Source: CAD feature listing. Evaluate the final solid. Frame: model axes, mm. A direction names the side the tool comes from. Round coordinates to 2 decimals unless told otherwise and drop trailing zeros. Loops run counter-clockwise (first coordinate to the right, second up) from the corner with the lowest first, then second, coordinate; pieces in that order, holes last. Notation, with made-up numbers: M 6,10.5 L 28,10.5 A27 cw 28,36.5 Z; hole C -35.75,80.5 d8. An arc over 180 degrees is marked long. One line per item, written item: value.
Autodesk Inventor part; units mm, degrees
ref_plane "Work Plane1" through (33.575, 0, 0) normal (0, 0, -1) x (1, 0, 0)
ref_plane "YZ Plane" through (0, 0, 0) normal (1, 0, 0) x (0, 1, 0)
ref_plane "XZ Plane" through (0, 0, 0) normal (0, 1, 0) x (-1, 0, 0)
sketch "Sketch1" plane through (0, 0, 0) normal (0, 0, 1) x (1, 0, 0)
  line L0 (0, 0) -> (10, 0)
  line L1 (10, 0) -> (10, 1.5)
  line L2 (10, 1.5) -> (2.65, 1.5)
  line L3 (2.65, 1.5) -> (2.3433, 1.5)
  line L4 (2.3433, 1.5) -> (1.65, 1.5)
  line L5 (1.65, 1.5) -> (0.35, 2.8)
  line L6 (0.35, 2.8) -> (0, 2.8)
  line L7 (0, 2.8) -> (0, 0)
  line L8 (2.65, 1.5) -> (1.65, 1.5) construction
  line L9 (-2, 0) -> (12, 0)
  line L10 (0, 3.36) -> (0, -0.56)
  dimension "d0" = 10
  dimension "d1" = 45
  dimension "d2" = 0.3067
  dimension "d3" = 7.35
  dimension "d4" = 1.65
  dimension "d5" = 3
  dimension "d6" = 3
  dimension "d7" = 5.6
revolve "Body" add sketch "Sketch1" angle 360 about axis through (0, 0, 0) along (1, 0, 0)
sketch "Sketch2" plane through (0, 0, 0) normal (-1, 0, 0) x (0, 0, 1)
  line L0 (2.8, -0.4) -> (-2.8, -0.4)
  line L1 (-2.8, -0.4) -> (-2.8, 0.4)
  line L2 (-2.8, 0.4) -> (2.8, 0.4)
  line L3 (2.8, 0.4) -> (2.8, -0.4)
  line L4 (0, 0.4) -> (0, -0.4) construction
  line L5 (-2.8, 0) -> (2.8, 0) construction
  line L6 (0, 2.8) -> (0, 0)
  dimension "d15" = 0.8
  dimension "d16" = 5.6
extrude "Slot" cut sketch "Sketch2" against normal blind 0.85
thread "Thread"
chamfer "Chamfer1" distance 0.3067 distance2 0.1534 1 edges at (10, -1.5, 0) measured on face at (10, 0.263, 0.1197)
ref_plane "Work Plane1" through (33.575, 0, 0) normal (0, 0, -1) x (1, 0, 0)
equation "\"d0\" = NLG"
equation "\"d1\" = 0.5 * SEWI"
equation "\"d2\" = GAL"
equation "\"d3\" = GEL"
equation "\"d4\" = KOH"
equation "\"d5\" = BDM"
equation "\"d6\" = GD"
equation "\"d7\" = KOD"
equation "\"d15\" = SBR"
equation "\"d16\" = KOD"
equation "\"d8\" = STI"
equation "\"d10\" = GEL"
equation "\"d12\" = -0.5 * SPD + 0.5 * GD"
equation "\"d13\" = 0.5 * GAL"
equation "\"NLG\" = 10"
equation "\"GAL\" = 0.61345 * PTC"
equation "\"GEL\" = 7.35"
equation "\"KOH\" = 1.65"
equation "\"KOD\" = 5.6"
equation "\"SEWI\" = 90deg"
equation "\"BDM\" = NND"
equation "\"GD\" = NND"
equation "\"SBR\" = 0.8"
equation "\"STI\" = 0.85"
equation "\"SPD\" = NND - 1.2269 * PTC"
equation "\"GUL\" = 0.61345 * PTC"
equation "\"PTC\" = 0.5"
equation "\"EPV\" = 3.15"
equation "\"THREADDIA\" = 3"
equation "\"TOA\" = 30deg"
equation "\"NND\" = 3"
equation "\"GD1\" = THREADDIA - 1.2269 * PTC"
properties part number "DIN 963 - M3 x 10" material "Steel, Mild"
1. Section query A-A (y = 0). Return the cut outline in (x, z).
Report:
outline: M 0.85,-2.3 L 1.65,-1.5 L 9.85,-1.5 L 10,-1.19 L 10,1.19 L 9.85,1.5 L 1.65,1.5 L 0.85,2.3 Z
2. Section query C-C (x = 4.25). Return the cut outline in (y, z), and give its area (3 significant figures).
Report:
outline: C 0,0 d3
area: 7.07 mm2
3. Reachability of faces 1 (the face through (0, 1, 0)), 2 (the face through (0.4, -0.4, 0)), 3 (the face through (5.69, -1.5, -0.07)) from +Z, -Z, +X, -X, +Y, -Y: full face, straight path, thin tool, end or side. Return the list, or none.
Report:
face 1: +Z, -Z, -X, +Y, -Y
face 2: +Z, -Z, -X
face 3: +X
4. Pin query (flat end, axial travel): pin 1 (2 mm diameter, centred on x = 4, z = -2, fed in from -Y); pin 2 (1 mm diameter, centred on x = 2.5, y = 0, fed in from +Z); pin 3 (3 mm diameter, centred on x = 4, z = -1.5, fed in from -Y). Return the tip coordinate at first contact, or that it passes through.
Report:
pin 1: stops at y = -1.12
pin 2: stops at z = 1.5
pin 3: stops at y = -1.5
5. Ray query, line 1 (X direction, y = 0, z = 0.9); line 2 (Z direction, x = 9.75, y = 0.6); line 3 (Y direction, x = 1.75, z = -0.9). Return the intervals inside material, ascending. Write a range as [from, to].
Report:
line 1: x = [0.85, 10]
line 2: z = [-1.37, 1.37]
line 3: y = [-1.2, 1.2]
6. Section query B-B (z = 0). Return the cut outline in (x, y).
Report:
outline: M 0,-2.8 L 0.35,-2.8 L 1.65,-1.5 L 9.85,-1.5 L 10,-1.19 L 10,1.19 L 9.85,1.5 L 1.65,1.5 L 0.35,2.8 L 0,2.8 L 0,0.4 L 0.85,0.4 L 0.85,-0.4 L 0,-0.4 Z
